Input: part model. Units: mm. Frame: model coordinates. Round coordinates to 2 decimals unless told otherwise and drop trailing zeros. Order: outer loops, then holes, each group sorted by start corner. A loop starts at its lowest first (then second) coordinate and runs counter-clockwise, first axis right, second up.
Item 1: First-contact query: pin 1 (3 mm diameter, centred on y = 3.5, z = 3, fed in from +X); pin 2 (5 mm diameter, centred on y = 2.5, z = 8, fed in from -X); pin 3 (12 mm diameter, centred on x = 28, z = -4.5, fed in from +Y); pin 4 (1.5 mm diameter, centred on y = 8, z = -6.5, fed in from +X). Flat tips, straight axial feed; report the tip coordinate or a pass-through.
Item 2: Cut plane C-C on y = 2. Output: boundary loops of the cut face in (x, z), then the cut area to 3 significant figures.
Item 3: Cut plane A-A on x = 11.5. Output: boundary loops of the cut face in (y, z).
Item 4: Line query: L1, parallel to X at y = 2.7, z = 0; L2, parallel to Z at x = -14, y = 4.75; L3, parallel to X at y = 3.5, z = -1.25. Output: solid intervals per line, ascending.
Item 5: Cut plane D-D on y = 6.75. Output: boundary loops of the cut face in (x, z), then the cut area to 3 significant figures.
Item 6: Cut plane B-B on z = 0. Output: boundary loops of the cut face in (x, y).
```python
from build123d import *

# Parameters (mm, degrees)
BOSS_EXTRUDE1_DEPTH = 5
CUT_EXTRUDE1_DEPTH  = 62.032778079
SKETCH3_R           = 5
BOSS_EXTRUDE2_DEPTH = 5
SKETCH4_R           = 5
CUT_EXTRUDE2_DEPTH  = 62.032778079


with BuildPart() as part:
    # Sketch1 → Boss-Extrude1 (new body)
    with BuildSketch(Plane(origin=(0, 0, 0), x_dir=(1, 0, 0), z_dir=(0, 1, 0))):
        with BuildLine():
            Line((-50, 10), (50, 10))
            ThreePointArc((50, 10), (60, 0), (50, -10))
            Line((50, -10), (-50, -10))
            ThreePointArc((-50, -10), (-60, 0), (-50, 10))
        make_face()
    extrude(amount=BOSS_EXTRUDE1_DEPTH)

    # Sketch2 → Cut-Extrude1 (cut, through all)
    with BuildSketch(Plane(origin=(0, 5, 0), x_dir=(1, 0, 0), z_dir=(0, 1, 0))):
        with BuildLine():
            Line((-35, 5), (35, 5))
            ThreePointArc((35, 5), (40, 0), (35, -5))
            Line((35, -5), (-35, -5))
            ThreePointArc((-35, -5), (-40, 0), (-35, 5))
        make_face()
    extrude(amount=-CUT_EXTRUDE1_DEPTH, mode=Mode.SUBTRACT)

    # Sketch3 → Boss-Extrude2 (add)
    with BuildSketch(Plane(origin=(0, 5, 0), x_dir=(1, 0, 0), z_dir=(0, 1, 0))):
        with Locations(Location((50, 0, 0), (0, 0, 270))):
            Circle(SKETCH3_R)
    extrude(amount=BOSS_EXTRUDE2_DEPTH)

    # Sketch4 → Cut-Extrude2 (cut, through all)
    with BuildSketch(Plane(origin=(0, 5, 0), x_dir=(1, 0, 0), z_dir=(0, 1, 0))):
        with Locations(Location((-50, 0, 0), (0, 0, 270))):
            Circle(SKETCH4_R)
    extrude(amount=-CUT_EXTRUDE2_DEPTH, mode=Mode.SUBTRACT)


solid = part.part
```
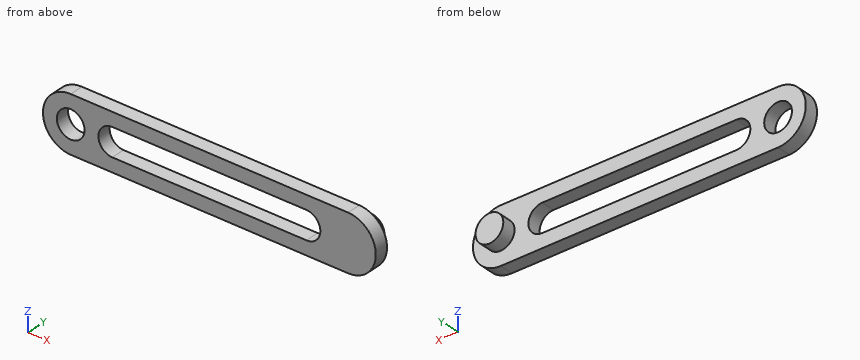
From the geometry:
1. pin 1: stops at x = 59.89
1. pin 2: stops at x = -58.35
1. pin 3: stops at y = 5
1. pin 4: passes through
2. outline: (-50, -10) - (50, -10) arc R10 ccw to (50, 10) - (-50, 10) arc R10 ccw to start; hole circle Ø10 at (-50, 0); hole (-35, -5) - (35, -5) arc R5 ccw to (35, 5) - (-35, 5) arc R5 ccw to start
2. area: 1,460 mm2
3. outline: (0, -10) - (5, -10) - (5, -5) - (0, -5) - close; (0, 5) - (5, 5) - (5, 10) - (0, 10) - close
4. L1: x = -60 to -55, -45 to -40, 40 to 60
4. L2: z = -10 to -5, 5 to 10
4. L3: x = -59.92 to -54.84, -45.16 to -39.84, 39.84 to 59.92
5. outline: circle Ø10 at (50, 0)
5. area: 78.5 mm2
6. outline: (-60, 0) - (-55, 0) - (-55, 5) - (-60, 5) - close; (-45, 0) - (-40, 0) - (-40, 5) - (-45, 5) - close; (40, 0) - (60, 0) - (60, 5) - (55, 5) - (55, 10) - (45, 10) - (45, 5) - (40, 5) - close
